Source: CAD feature listing. Evaluate the final solid. Frame: model axes, mm. A direction names the side the tool comes from. Coordinates: 2 decimals unless noted, no trailing zeros. Write each loop counter-clockwise with the first axis right and the second up, starting at its lowest first coordinate (ties: lowest second). Pieces come first, ordered by that corner, then holes. Notation, with made-up numbers: (17.5, 23.5) -> (65.5, 23.5) arc R17 ccw to (65.5, 43.5) -> close; hole circle Ø5 at (46.25, 8). An arc over 180 degrees is marked (long way). Write item = value, one per line.
Autodesk Fusion 360 part; units mm, degrees
sketch "Sketch1" plane through (0, 0, 0) normal (0, 1, 0) x (1, 0, 0)
  circle A0 centre (-29.052, 0) radius 8
  circle A1 centre (26.948, 0) radius 8
  line L0 (-29, -17.9738) -> (27, -17.9738)
  line L1 (-29, 17.9738) -> (27, 17.9738)
  arc A2 (25.9777, -17.9738) -> (25.9777, 17.9738) centre (26.948, 0) ccw
  arc A3 (-28.0816, 17.9738) -> (-28.0816, -17.9738) centre (-29.052, 0) ccw
  dimension "d1" = 56
  dimension "d2" = 16
  dimension "d3" = 16
  dimension "d5" = 36
  dimension "d6" = 36
extrude "Extrude1" add sketch "Sketch1" along normal blind 8
sketch "Sketch2" plane through (0, 8, 0) normal (0, 1, 0) x (-1, 0, 0)
  circle A0 centre (-26.948, 0) radius 8
  circle A1 centre (29.052, 0) radius 8
  arc A2 (28.0816, -17.9738) -> (28.0816, 17.9738) centre (29.052, 0) ccw
  line L0 (28.0816, 17.9738) -> (-25.9777, 17.9738)
  arc A3 (-25.9777, 17.9738) -> (-25.9777, -17.9738) centre (-26.948, 0) ccw
  line L1 (-25.9777, -17.9738) -> (28.0816, -17.9738)
  line L2 (21.1928, -17.9738) -> (-18.8072, -17.9738)
  line L3 (-18.8072, -17.9738) -> (-18.8072, -7.9738)
  line L4 (-18.8072, -7.9738) -> (21.1928, -7.9738)
  line L5 (21.1928, -7.9738) -> (21.1928, -17.9738)
  dimension "d9" = 40
  dimension "d10" = 10
  dimension "d11" = 40
  dimension "d12" = 40
  dimension "d13" = 10
extrude "Extrude2" add sketch "Sketch2" along normal blind 32 contours L1 L2 L3 L4 L5
sketch "Sketch3" plane through (0, 0, -17.9738) normal (0, 0, -1) x (-1, 0, 0)
  line L0 (-25.9777, 0) -> (28.0816, 0)
  line L1 (28.0816, 0) -> (28.0816, 8)
  line L2 (28.0816, 8) -> (21.1928, 8)
  line L3 (21.1928, 8) -> (21.1928, 40)
  line L4 (21.1928, 40) -> (-18.8072, 40)
  line L5 (-18.8072, 40) -> (-18.8072, 8)
  line L6 (-18.8072, 8) -> (-25.9777, 8)
  line L7 (-25.9777, 8) -> (-25.9777, 0)
  line L8 (-18.8072, 40) -> (21.1928, 40)
  line L9 (21.1928, 40) -> (21.1928, 30)
  line L10 (21.1928, 30) -> (-18.8072, 30)
  line L11 (-18.8072, 30) -> (-18.8072, 40)
  dimension "d16" = 10
extrude "Extrude3" add sketch "Sketch3" along normal blind 32 contours L3 L4 L5 L8 L9 L10 L11
sketch "Sketch4" plane through (0, 40, 0) normal (0, 1, 0) x (-1, 0, 0)
  line L0 (21.1928, -7.9738) -> (-18.8072, -7.9738)
  line L1 (-18.8072, -7.9738) -> (-18.8072, -49.9738)
  line L2 (-18.8072, -49.9738) -> (21.1928, -49.9738)
  line L3 (21.1928, -49.9738) -> (21.1928, -7.9738)
  line L4 (21.1928, -28.6563) -> (15.1408, -50.6921)
  line L5 (-19.0097, -28.6563) -> (-12.9578, -50.6921)
extrude "Extrude4" cut sketch "Sketch4" against normal blind 20 contours L2 L3 L4
sketch "Sketch5" plane through (0, 40, 0) normal (0, 1, 0) x (-1, 0, 0)
  line L0 (15.3381, -49.9738) -> (21.1928, -28.6563)
  line L1 (21.1928, -28.6563) -> (21.1928, -7.9738)
  line L2 (21.1928, -7.9738) -> (-18.8072, -7.9738)
  line L3 (-18.8072, -7.9738) -> (-18.8072, -49.9738)
  line L4 (-18.8072, -49.9738) -> (15.3381, -49.9738)
  line L5 (1.1928, 40.1018) -> (1.1928, -51.5866)
  line L6 (-12.9526, -49.9738) -> (-18.8072, -28.6563)
extrude "Extrude5" cut sketch "Sketch5" against normal blind 30 contours L3 L4 L6
sketch "Sketch6" plane through (0, 40, 0) normal (0, 1, 0) x (-1, 0, 0)
  line L0 (-18.8072, -28.6563) -> (-12.9526, -49.9738)
  line L1 (-12.9526, -49.9738) -> (15.3381, -49.9738)
  line L2 (15.3381, -49.9738) -> (21.1928, -28.6563)
  line L3 (21.1928, -28.6563) -> (21.1928, -7.9738)
  line L4 (21.1928, -7.9738) -> (-18.8072, -7.9738)
  line L5 (-18.8072, -7.9738) -> (-18.8072, -28.6563)
  circle A0 centre (1.1928, -49.9738) radius 15
  circle A1 centre (1.1928, -49.9738) radius 10
  dimension "d23" = 30
  dimension "d24" = 20
extrude "Extrude6" add sketch "Sketch6" along normal blind 10 contours L0 L1 L2 A0 A1 | L0 L1 L2 A0 A1
extrude "Extrude7" add 1 faces at (1.7657, 40, -62.9484) along direction (0, -1, 0) blind 10
extrude "Extrude8" cut 1 faces at (-2.0826, 40, -45.7415) along direction (0, -1, 0) blind 45
sketch "Sketch7" plane through (0, 8, 0) normal (0, 1, 0) x (-1, 0, 0)
  line L0 (-18.8072, -17.9738) -> (-18.8072, -7.9738)
  line L1 (-18.8072, -7.9738) -> (21.1928, -7.9738)
  line L2 (21.1928, -7.9738) -> (21.1928, -17.9738)
  line L3 (21.1928, -17.9738) -> (28.0816, -17.9738)
  arc A0 (28.0816, -17.9738) -> (28.0816, 17.9738) centre (29.052, 0) ccw
  line L4 (28.0816, 17.9738) -> (-25.9777, 17.9738)
  arc A1 (-25.9777, 17.9738) -> (-25.9777, -17.9738) centre (-26.948, 0) ccw
  line L5 (-25.9777, -17.9738) -> (-18.8072, -17.9738)
  circle A2 centre (29.052, 0) radius 8
  circle A3 centre (-26.948, 0) radius 8
  line L6 (6.0956, -7.9738) -> (-5.9044, -7.9738)
  line L7 (-5.9044, -7.9738) -> (-5.9044, 17.6922)
  line L8 (-5.9044, 17.6922) -> (6.0956, 17.6922)
  line L9 (6.0956, 17.6922) -> (6.0956, -7.9738)
  dimension "d31" = 12
extrude "Extrude9" add sketch "Sketch7" along normal blind 32 contours L1 L6 L7 L8 L9
sketch "Sketch8" plane through (5.9044, 0, 0) normal (1, 0, 0) x (0, 0, -1)
  line L0 (-17.6922, 8) -> (7.9738, 8)
  line L1 (7.9738, 8) -> (7.9738, 40)
  line L2 (7.9738, 40) -> (-17.6922, 40)
  line L3 (-17.6922, 40) -> (-17.6922, 8)
  line L4 (-17.6922, 8) -> (7.9738, 40)
extrude "Extrude10" cut sketch "Sketch8" against normal blind 55 contours L2 L3 L4
1) Material intervals for probe 1 along X at (y, z) = (5.5, 0); probe 2 along X at (y, z) = (3, -5); probe 3 along Y at (x, z) = (36.5, -3), sorted ascending. Write a range as [from, to].
Answer block:
probe_1 = [-47.05, -37.05], [-21.05, 18.95], [34.95, 44.95]
probe_2 = [-46.34, -35.3], [-22.81, 20.7], [33.19, 44.24]
probe_3 = [0, 8]
2) Cut plane D-D, the plane y = 33. Output: boundary loops of the cut face in (x, z), and give its area (3 significant figures).
Answer block:
outline = (-21.19, -28.66) -> (-16, -47.57) arc R15 ccw (long way) to (13.61, -47.57) -> (18.81, -28.66) -> (18.81, -7.97) -> (5.9, -7.97) -> (5.9, -2.36) -> (-6.1, -2.36) -> (-6.1, -7.97) -> (-21.19, -7.97) -> close; hole circle Ø20 at (-1.19, -49.97)
area = 1,660 mm2
3) Cut plane A-A, the plane x = -1.5. Output: boundary loops of the cut face in (y, z).
Answer block:
outline = (0, -17.97) -> (30, -17.97) -> (30, -39.98) -> (50, -39.98) -> (50, -34.98) -> (40, -34.98) -> (40, -7.97) -> (8, 17.69) -> (8, 17.97) -> (0, 17.97) -> close; (30, -64.97) -> (50, -64.97) -> (50, -59.97) -> (30, -59.97) -> close
4) First-contact query: pin 1 Ø16.5 at (y, z) = (30, -16.5) entering from -X; pin 2 Ø2 at (x, y) = (33.5, 10.5) entering from -Z; pin 3 Ø2 at (x, y) = (-14, 40) entering from +Z; pin 4 Ø11 at (x, z) = (-19.5, -4.5) entering from +Y. Flat tips, straight axial feed; report the tip coordinate or a pass-through.
Answer block:
pin_1 = -21.19
pin_2 = through
pin_3 = -7.97
pin_4 = 40
5) Reachability of faces 1 (the flat face through (-21.193, 27, -16)), 2 (the flat face through (18.807, 28, -16)), 3 (the cylindrical face through (0.76, 42.082, -64.846)), 4 (the flat face through (-14, 24, -7.974)) from +Z, -Z, +X, -X, +Y, -Y: full face, straight path, thin tool, end or side. Return the list, or none.
Answer block:
face_1 = +Z, -Z, -X, +Y
face_2 = +Z, -Z, +X, +Y
face_3 = +Y
face_4 = +Z, -X, +Y
6) Cut plane C-C, the plane x = -19.5. Output: boundary loops of the cut face in (y, z).
Answer block:
outline = (0, -17.97) -> (30, -17.97) -> (30, -34.82) -> (40, -34.82) -> (40, -7.97) -> (8, -7.97) -> (8, 17.97) -> (0, 17.97) -> close
7) Cut plane B-B, the plane z = 0. Output: boundary loops of the cut face in (x, y).
Answer block:
outline = (-47.05, 0) -> (-37.05, 0) -> (-37.05, 8) -> (-47.05, 8) -> close; (-21.05, 0) -> (18.95, 0) -> (18.95, 8) -> (5.9, 8) -> (5.9, 30.06) -> (-6.1, 30.06) -> (-6.1, 8) -> (-21.05, 8) -> close; (34.95, 0) -> (44.95, 0) -> (44.95, 8) -> (34.95, 8) -> close
8) Pull-direction query (Z, two-part tool) for faces 5 (the flat face through (9, 8, 4)), 6 (the cylindrical face through (0.11, 40.14, -40.06)), 7 (the flat face through (12, 24, -7.974)); classes: +Z half, -Z half, draft (parallel to the pull), parting line (faces both ways), or undercut.
Answer block:
face_5 = draft
face_6 = undercut
face_7 = +Z half
